Input: part model. Units: mm. Frame: model coordinates. Coordinates: 2 decimals unless noted, no trailing zeros. Loops run counter-clockwise (first coordinate to the right, second up) from the corner with the lowest first, then second, coordinate; pieces in that order, holes last.
```python
from build123d import *

# Parameters (mm, degrees)
SKETCH_1_W                  = 65
SKETCH_1_H                  = 59
EXTRUDE_1_DEPTH             = 27
SKETCH_2_R                  = 2.5
CUT_EXTRUDE_1_DEPTH         = 27
PATTERN_LINEAR_1_COUNT      = 2
PATTERN_LINEAR_1_PITCH      = 50
PATTERN_LINEAR_1_COUNT_DIR2 = 2
PATTERN_LINEAR_1_PITCH_DIR2 = 20
SKETCH_3_R                  = 1.65
CUT_EXTRUDE_2_DEPTH         = 27
PATTERN_LINEAR_2_COUNT      = 2
PATTERN_LINEAR_2_PITCH      = 30
PATTERN_LINEAR_2_COUNT_DIR2 = 2
PATTERN_LINEAR_2_PITCH_DIR2 = 30


with BuildPart() as part:
    # Эскиз1 → Бобышка-Вытянуть1 (new body)
    with BuildSketch(Plane.XY):
        Rectangle(SKETCH_1_W, SKETCH_1_H)
    extrude(amount=EXTRUDE_1_DEPTH)

    # Эскиз2 → Вырез-Вытянуть1 (cut)
    with BuildSketch(Plane.XY.offset(27)):
        with Locations((-25, 20.5)):
            Circle(SKETCH_2_R)
    cut_extrude_1 = extrude(amount=-CUT_EXTRUDE_1_DEPTH, mode=Mode.SUBTRACT)

    # Линейный массив1: Cut-Extrude 1 2 × 2
    with Locations(*[(i * PATTERN_LINEAR_1_PITCH, -j * PATTERN_LINEAR_1_PITCH_DIR2, 0) for i in range(PATTERN_LINEAR_1_COUNT) for j in range(PATTERN_LINEAR_1_COUNT_DIR2) if (i, j) != (0, 0)]):
        add(cut_extrude_1, mode=Mode.SUBTRACT)

    # Эскиз3 → Вырез-Вытянуть2 (cut)
    with BuildSketch(Plane.XY.offset(27)):
        with Locations((-15, 15)):
            Circle(SKETCH_3_R)
    cut_extrude_2 = extrude(amount=-CUT_EXTRUDE_2_DEPTH, mode=Mode.SUBTRACT)

    # Линейный массив2: Cut-Extrude 2 2 × 2
    with Locations(*[(i * PATTERN_LINEAR_2_PITCH, -j * PATTERN_LINEAR_2_PITCH_DIR2, 0) for i in range(PATTERN_LINEAR_2_COUNT) for j in range(PATTERN_LINEAR_2_COUNT_DIR2) if (i, j) != (0, 0)]):
        add(cut_extrude_2, mode=Mode.SUBTRACT)


solid = part.part
```
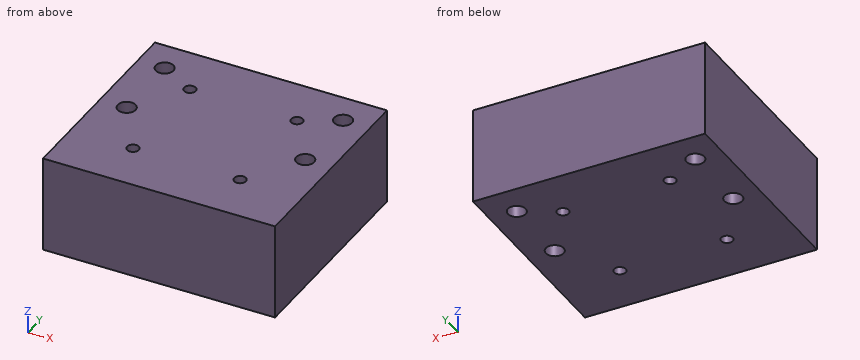
Item 1: Line query: L1, parallel to Y at x = -25, z = 19; L2, parallel to Y at x = 15, z = 19.5; L3, parallel to X at y = 18.5, z = 3. Output: solid intervals per line, ascending.
Result:
L1: y = -29.5 to -2, 3 to 18, 23 to 29.5
L2: y = -29.5 to -16.65, -13.35 to 13.35, 16.65 to 29.5
L3: x = -32.5 to -26.5, -23.5 to 23.5, 26.5 to 32.5
Item 2: Section query A-A (x = -25). Output: boundary loops of the cut face in (y, z).
Result:
outline: (-29.5, 0) - (-2, 0) - (-2, 27) - (-29.5, 27) - close; (3, 0) - (18, 0) - (18, 27) - (3, 27) - close; (23, 0) - (29.5, 0) - (29.5, 27) - (23, 27) - close
Item 3: Contact query for a flat-ended pin moving along its axis: P1, Ø1, axis at x = -25.5, y = -15, coming from the -Z side. Output: stop coordinate, or through.
Result:
P1: stops at z = 0
Item 4: Section query B-B (z = 10.5). Count the separate pieces of the cut face and the enclosed holes in it, then the cut area to 3 significant figures.
Result:
separate pieces: 1
enclosed holes: 8
area: 3,720 mm2
Item 5: Section query C-C (y = 0.5). Output: boundary loops of the cut face in (x, z).
Result:
outline: (-32.5, 0) - (-27.5, 0) - (-27.5, 27) - (-32.5, 27) - close; (-22.5, 0) - (22.5, 0) - (22.5, 27) - (-22.5, 27) - close; (27.5, 0) - (32.5, 0) - (32.5, 27) - (27.5, 27) - close
